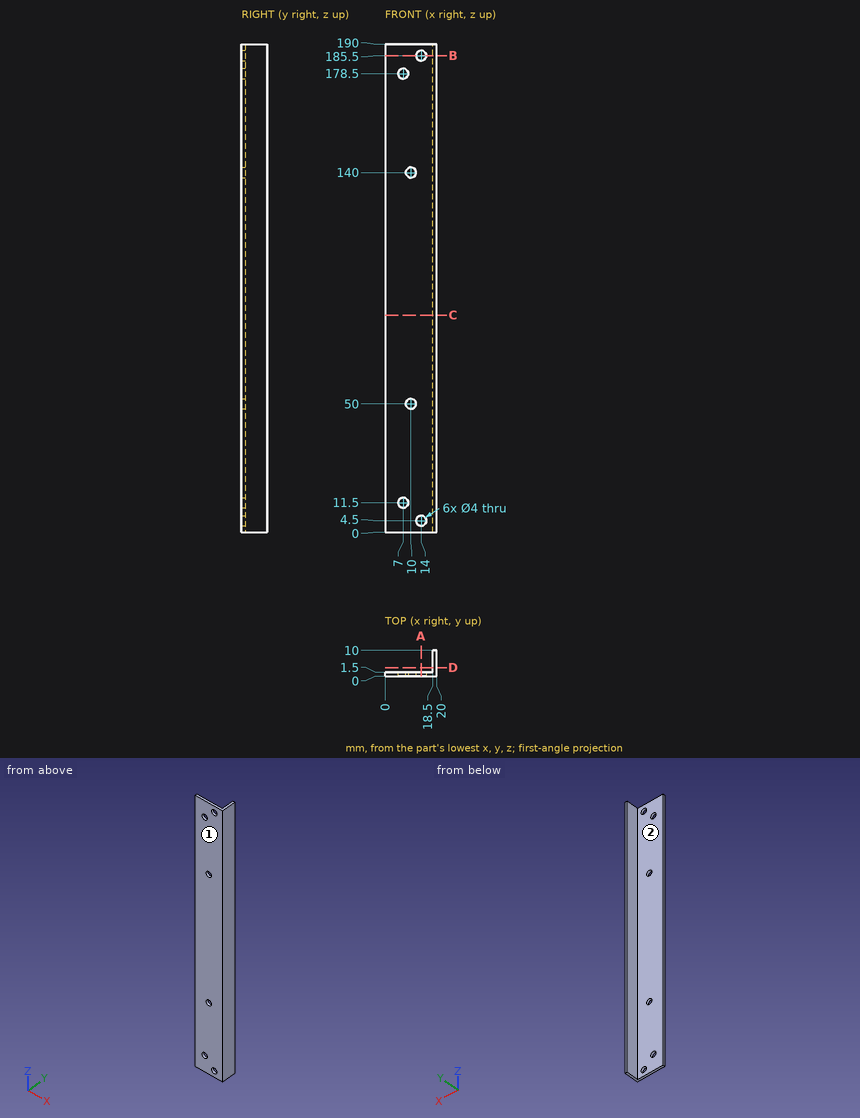
Print and shaded views of the part. All mm, measured from the part's lowest x, y and z. A direction names the side the tool comes from. Coordinates: 2 decimals unless noted, no trailing zeros. Loops run counter-clockwise (first coordinate to the right, second up) from the corner with the lowest first, then second, coordinate; pieces in that order, holes last. Notation, with made-up numbers: (-31, 8.5) - (26, 8.5) arc R24 cw to (26, 35.5) - close; hole circle Ø5 at (33, 67.5). An arc over 180 degrees is marked (long way). Write item = value, one per line. Start each with the question number.
Item 1: Wall check: L1, parallel to Z at x = 10, y = 0.45; L2, parallel to Z at x = 14, y = 1.1; L3, parallel to X at y = 1.1, z = 178.5. Give the ranges that are in metal, low to high. Write a range as from..to.
Item 2: Flat gauge pins, fed straight in: pin 1 Ø4.5 at (x, z) = (10, 50) entering from -Y; pin 2 Ø2 at (x, y) = (8, 3) entering from +Z; pin 3 Ø4 at (y, z) = (6.5, 90) entering from -X; pin 4 Ø4.5 at (x, z) = (7, 178.5) entering from +Y. Where does each tip first touch, or does it go through?
Item 3: Cut at A-A, the plane x = 14. Give the cut face in (y, z), and give its area (3 significant figures).
Item 4: Cut at C-C, the plane z = 84.5. Give the cut face in (x, y).
Item 5: Cut at D-D, the plane y = 3.25. Give the cut face in (x, z), and give its area (3 significant figures).
Item 6: 3-axis set-ups, long thin cutter, end or side, ignore diameter. For the marked faces 1 and 2: which of +Z, -Z, +X, -X, +Y, -Y reach the whole face in a straight line?
Item 7: Cut at B-B, the plane z = 185.5. Give the cut face in (x, y).
The answers:
q1.L1 = 0..48, 52..138, 142..190
q1.L2 = 0..2.5, 6.5..183.5, 187.5..190
q1.L3 = 0..5, 9..20
q2.pin_1 = 0
q2.pin_2 = through
q2.pin_3 = 18.5
q2.pin_4 = 1.5
q3.outline = (0, 0) - (1.5, 0) - (1.5, 2.5) - (0, 2.5) - close; (0, 6.5) - (1.5, 6.5) - (1.5, 183.5) - (0, 183.5) - close; (0, 187.5) - (1.5, 187.5) - (1.5, 190) - (0, 190) - close
q3.area = 273 mm2
q4.outline = (0, 0) - (20, 0) - (20, 10) - (18.5, 10) - (18.5, 1.5) - (0, 1.5) - close
q5.outline = (18.5, 0) - (20, 0) - (20, 190) - (18.5, 190) - close
q5.area = 285 mm2
q6.face_1 = +Z, -Z, +X, -X, -Y
q6.face_2 = +Z, -Z, -X, +Y
q7.outline = (0, 0) - (12, 0) - (12, 1.5) - (0, 1.5) - close; (16, 0) - (20, 0) - (20, 10) - (18.5, 10) - (18.5, 1.5) - (16, 1.5) - close
